Autodesk Inventor part; units mm, degrees
ref_plane "YZ Plane" through (0, 0, 0) normal (1, 0, 0) x (0, 1, 0)
ref_plane "XZ Plane" through (0, 0, 0) normal (0, 1, 0) x (-1, 0, 0)
ref_plane "XY Plane" through (0, 0, 0) normal (0, 0, 1) x (1, 0, 0)
sketch "Sketch1" plane through (0, 0, 0) normal (0, 1, 0) x (-1, 0, 0)
  line L0 (25, -5) -> (-25, -5)
  line L1 (-25, -5) -> (-25, 5)
  line L2 (-25, 5) -> (25, 5)
  line L3 (25, 5) -> (25, -5)
  line L4 (25, -5) -> (-25, 5) construction
  line L5 (-25, -5) -> (25, 5) construction
  point P0 (0, 0)
  dimension "d0" = 10
  dimension "d1" = 50
extrude "Extrusion1" add sketch "Sketch1" along normal blind 2
sketch "Sketch2" plane through (0, 2, 0) normal (0, 1, 0) x (1, 0, 0)
  line L0 (-25, -5) -> (25, -5)
  line L1 (25, -5) -> (25, 5)
  line L2 (25, 5) -> (-25, 5)
  line L3 (-25, 5) -> (-25, -5)
  line L4 (-25, 0) -> (25, 0)
  line L5 (0, 5) -> (0, -5)
  point P0 (0, 0)
  point P1 (-18, 0)
  point P2 (18, 0)
  dimension "d11" = 18
  dimension "d12" = 18
hole "Hole1" at (-18, 2, 0) at (18, 2, 0) direction (0, -1, 0) diameter 1.778 end through all
sketch "Sketch3" plane through (0, 2, 0) normal (0, 1, 0) x (1, 0, 0)
  circle A0 centre (-18, 0) radius 0.889
  circle A1 centre (18, 0) radius 0.889
  line L0 (-25, -5) -> (25, -5)
  line L1 (25, -5) -> (25, 5)
  line L2 (25, 5) -> (-25, 5)
  line L3 (-25, 5) -> (-25, -5)
  line L4 (-25, 0) -> (25, 0) construction
  line L5 (0, 5) -> (0, -5) construction
  point P0 (0, 0)
  point P1 (14, 0)
  point P2 (-14, 0)
  point P3 (-10, 0)
  point P4 (-6, 0)
  point P5 (-2, 0)
  point P6 (2, 0)
  point P7 (6, 0)
  point P8 (10, 0)
  dimension "d21" = 4
  dimension "d22" = 4
  dimension "d23" = 4
  dimension "d24" = 2
  dimension "d25" = 2
  dimension "d26" = 4
  dimension "d27" = 4
  dimension "d28" = 4
hole "Hole2" at (14, 2, 0) at (-14, 2, 0) at (-10, 2, 0) at (-6, 2, 0) at (-2, 2, 0) at (2, 2, 0) at (6, 2, 0) at (10, 2, 0) direction (0, -1, 0) diameter 1.778 end through all
sketch "Sketch4" plane through (0, 2, 0) normal (0, 1, 0) x (1, 0, 0)
  circle A0 centre (6, 0) radius 0.889
  circle A1 centre (-2, 0) radius 0.889
  circle A2 centre (-10, 0) radius 0.889
  circle A3 centre (14, 0) radius 0.889
  circle A4 centre (-14, 0) radius 0.889
  circle A5 centre (-6, 0) radius 0.889
  circle A6 centre (2, 0) radius 0.889
  circle A7 centre (10, 0) radius 0.889
  circle A8 centre (-18, 0) radius 0.889
  circle A9 centre (18, 0) radius 0.889
  line L0 (-25, -5) -> (25, -5)
  line L1 (25, -5) -> (25, 5)
  line L2 (25, 5) -> (-25, 5)
  line L3 (-25, 5) -> (-25, -5)
  line L4 (-25, 0) -> (25, 0) construction
  point P0 (0, 0)
  point P1 (-22, -0.0247)
  point P2 (22, 0.138)
  dimension "d37" = 4
  dimension "d38" = 4
hole "Hole3" at (-22, 2, 0.0247) at (22, 2, -0.138) direction (0, -1, 0) diameter 2 end through all
properties part number "Busbar Copper"
Check sheet for the modelled part. Datum: model origin and axes. Units: mm. Coordinates: 2 decimals unless noted, no trailing zeros. Write each loop counter-clockwise with the first axis right and the second up, starting at its lowest first coordinate (ties: lowest second). Pieces come first, ordered by that corner, then holes. Notation, with made-up numbers: M 12,-16 L 41,-16 A30 cw 41,8 Z; hole C 54,75 d4. An arc over 180 degrees is marked long. Answer as CSV lines item,"result".
Q1. Mould release check, pull along X, two halves, no side actions. Record for faces 1 (the face through (0, 2, 0)), 2 (the face through (-5.13, 0.99, -0.19)), 3 (the face through (-25, 1, 0)), 4 (the face through (25, 1, 0)): released by +X, released by -X, zero draft, split by the parting line, or undercut.
Check result:
face 1,"zero draft"
face 2,"undercut"
face 3,"released by -X"
face 4,"released by +X"
Q2. Cross-section at A-A (y = 1.15). Count the separate pieces of the cut face and the enclosed holes in it, then the cut area to 3 significant figures.
Check result:
separate pieces,"1"
enclosed holes,"12"
area,"469 mm^2"
Q3. Material ranges on probe 1 along Z at (x, y) = (-10, 0.8), recorded low to high. Write a range as from..to.
Check result:
probe 1,"-5..-0.89, 0.89..5"
Q4. Cross-section at B-B (x = -10). Record the boundary of the cut face in (y, z), then the cut area to 3 significant figures.
Check result:
outline,"M 0,-5 L 2,-5 L 2,-0.89 L 0,-0.89 Z; M 0,0.89 L 2,0.89 L 2,5 L 0,5 Z"
area,"16.4 mm^2"
Q5. Go/stop test with a flat-tipped pin: pin 1 (1.4 mm diameter, centred on x = 2, z = 0, fed in from +Y). Record where the tip stops, or that it passes through.
Check result:
pin 1,"through"
Q6. Cross-section at C-C (x = -22). Record the boundary of the cut face in (y, z), then the cut area to 3 significant figures.
Check result:
outline,"M 0,-5 L 2,-5 L 2,-0.98 L 0,-0.98 Z; M 0,1.02 L 2,1.02 L 2,5 L 0,5 Z"
area,"16.0 mm^2"
